from build123d import *

# Parameters (mm, degrees)
SKETCH_1_W          = 42
SKETCH_1_H          = 5
EXTRUDE_1_DEPTH     = 18
SKETCH_2_R          = 1.55
CUT_EXTRUDE_1_DEPTH = 14.93
SKETCH_3_R          = 1.61
CUT_EXTRUDE_2_DEPTH = 28.771388154


with BuildPart() as part:
    # 草图1 → 凸台-拉伸1 (new body)
    with BuildSketch(Plane(origin=(0, 0, 0), x_dir=(1, 0, 0), z_dir=(0, 1, 0))):
        Rectangle(SKETCH_1_W, SKETCH_1_H)
    extrude(amount=EXTRUDE_1_DEPTH)

    # 草图2 → 切除-拉伸1 (cut)
    with BuildSketch(Plane.XY.offset(2.5)):
        with Locations((-18.995, 13.83)):
            Circle(SKETCH_2_R)
        with Locations((18.995, 13.83)):
            Circle(SKETCH_2_R)
    extrude(amount=-CUT_EXTRUDE_1_DEPTH, mode=Mode.SUBTRACT)

    # 草图3 → 切除-拉伸2 (cut, through all)
    with BuildSketch(Plane(origin=(0, 18, 0), x_dir=(1, 0, 0), z_dir=(0, 1, 0))):
        with Locations(Location((-11.345, 0, 0), (0, 0, 270))):
            Circle(SKETCH_3_R)
        with Locations(Location((11.345, 0, 0), (0, 0, 270))):
            Circle(SKETCH_3_R)
    extrude(amount=-CUT_EXTRUDE_2_DEPTH, mode=Mode.SUBTRACT)


solid = part.part
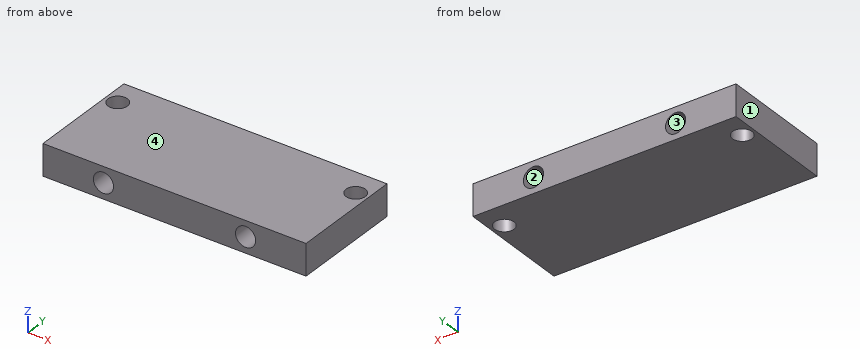
Check sheet for the modelled part. Datum: model origin and axes. Units: mm. Face numbers are marked on the shaded views. Coordinates: 2 decimals unless noted, no trailing zeros. Loops run counter-clockwise (first coordinate to the right, second up) from the corner with the lowest first, then second, coordinate; pieces in that order, holes last. Notation, with made-up numbers: (31, 59) -> (39, 59) arc R11 ccw to (39, 76) -> close; hole circle Ø5 at (-7.75, 17.5). An arc over 180 degrees is marked (long way). Write item = value, one per line. Start each with the question number.
1. Section check D-D on x = 18.5. Record the cut outline in (y, z), then the cut area to 3 significant figures.
2. Material ranges on line 1 (X direction, y = 1.25, z = 0) (3 decimals); line 2 (X direction, y = 8.5, z = -0.4); line 3 (X direction, y = 12.5, z = 0) (3 decimals), recorded low to high.
3. Section check B-B on y = 13.83. Record the cut outline in (x, z) (3 decimals).
4. Draft check along X on the marked faces 1, 2, 3 and 4. Enter one of: released by +X, released by -X, zero draft, split by the parting line, or undercut.
5. Section check C-C on z = 2. Record the cut outline in (x, y) (3 decimals).
6. Section check A-A on z = 0. Record the cut outline in (x, y) (3 decimals).
7. Depth check by flat-ended pin: P1, Ø2.5, axis at x = -11.345, z = 0, coming from the +Y side. Enter the tip coordinate at first touch or a pass-through.
Responses:
q1.outline = (0, -2.5) -> (12.36, -2.5) -> (12.36, 2.5) -> (0, 2.5) -> close; (15.3, -2.5) -> (18, -2.5) -> (18, 2.5) -> (15.3, 2.5) -> close
q1.area = 75.3 mm2
q2.line_1 = -21 to -12.955, -9.735 to 9.735, 12.955 to 21
q2.line_2 = -21 to -12.9, -9.79 to 9.79, 12.9 to 21
q2.line_3 = -21 to -19.791, -18.199 to -12.955, -9.735 to 9.735, 12.955 to 18.199, 19.791 to 21
q3.outline = (-21, -2.5) -> (-20.545, -2.5) -> (-20.545, 2.5) -> (-21, 2.5) -> close; (-17.445, -2.5) -> (17.445, -2.5) -> (17.445, 2.5) -> (-17.445, 2.5) -> close; (20.545, -2.5) -> (21, -2.5) -> (21, 2.5) -> (20.545, 2.5) -> close; hole circle Ø3.22 at (-11.345, 0); hole circle Ø3.22 at (11.345, 0)
q4.face_1 = released by -X
q4.face_2 = undercut
q4.face_3 = undercut
q4.face_4 = zero draft
q5.outline = (-21, 0) -> (21, 0) -> (21, 18) -> (-21, 18) -> close; hole circle Ø3.1 at (-18.995, 13.83); hole circle Ø3.1 at (18.995, 13.83)
q6.outline = (-21, 0) -> (-12.955, 0) -> (-12.955, 18) -> (-21, 18) -> close; (-9.735, 0) -> (9.735, 0) -> (9.735, 18) -> (-9.735, 18) -> close; (12.955, 0) -> (21, 0) -> (21, 18) -> (12.955, 18) -> close; hole circle Ø3.1 at (-18.995, 13.83); hole circle Ø3.1 at (18.995, 13.83)
q7.P1 = through
